Autodesk Inventor part; units mm, degrees
ref_plane "YZ Plane" through (0, 0, 0) normal (1, 0, 0) x (0, 1, 0)
ref_plane "XZ Plane" through (0, 0, 0) normal (0, 1, 0) x (-1, 0, 0)
ref_plane "XY Plane" through (0, 0, 0) normal (0, 0, 1) x (1, 0, 0)
sketch "Esquisse1" plane through (0, 0, 0) normal (0, 1, 0) x (-1, 0, 0)
  line L0 (25, 0) -> (125, 0)
  line L1 (150, -25) -> (150, -260)
  line L2 (125, -285) -> (25, -285)
  line L3 (0, -260) -> (0, -25)
  line L4 (20, 0) -> (20, -10) construction
  line L5 (20, -10) -> (0, -10) construction
  line L6 (150, 0) -> (0, -285) construction
  line L7 (150, -285) -> (0, 0) construction
  line L8 (75, 0) -> (75, -285) construction
  line L9 (150, -142.5) -> (0, -142.5) construction
  line L10 (30, -10) -> (120, -10)
  line L11 (130, -20) -> (130, -265)
  line L12 (120, -275) -> (30, -275)
  line L13 (20, -265) -> (20, -20)
  line L14 (130, -275) -> (150, -275) construction
  line L15 (130, -275) -> (130, -285) construction
  arc A0 (120, -275) -> (130, -265) centre (120, -265) ccw
  arc A1 (20, -265) -> (30, -275) centre (30, -265) ccw
  arc A2 (30, -10) -> (20, -20) centre (30, -20) ccw
  arc A3 (130, -20) -> (120, -10) centre (120, -20) ccw
  arc A4 (25, 0) -> (0, -25) centre (25, -25) ccw
  arc A5 (150, -25) -> (125, 0) centre (125, -25) ccw
  arc A6 (125, -285) -> (150, -260) centre (125, -260) ccw
  arc A7 (0, -260) -> (25, -285) centre (25, -260) ccw
  point P0 (150, -10)
  point P1 (148, 0)
  point P2 (0, -10)
  point P3 (10, 0)
  point P4 (0, -283)
  point P5 (2, -285)
  point P6 (140, -285)
  point P7 (150, -283)
  dimension "d0" = 150
  dimension "d5" = 20
  dimension "d11" = 10
  dimension "d13" = 10
  dimension "d14" = 265
  dimension "d15" = 25
extrude "Extrusion1" add sketch "Esquisse1" along normal blind 6
properties part number "top" material "Bois (cerisier)"
Geometry check sheet. Reference: the model listing, model coordinates, mm. A direction names the side the tool comes from. Round coordinates to 2 decimals unless told otherwise and drop trailing zeros. Write each loop counter-clockwise with the first axis right and the second up, starting at its lowest first coordinate (ties: lowest second). Pieces come first, ordered by that corner, then holes. Notation, with made-up numbers: (63.25, 20.5) -> (111.25, 20.5) arc R36 ccw to (111.25, 59.5) -> close; hole circle Ø3 at (-37.75, -29.75). An arc over 180 degrees is marked (long way). Put each result on its own line as item: value.
1) Release check for a two-part mould opening along X. For faces 1 (the face through (-19, 0, -142)), 2 (the face through (-23.01, 2.96, -272.15)), 3 (the face through (-142.871, 2.958, -277.482)) record: pulls with the +X half, pulls with the -X half, needs draft (parallel to the pull), parting line crosses it, or undercut.
Recorded:
face 1: needs draft
face 2: undercut
face 3: pulls with the -X half
2) Depth check by flat-ended pin: P1, Ø1, axis at y = 3.5, z = -33.5, coming from the +X side. Enter the tip coordinate at first touch or a pass-through.
Recorded:
P1: stops at x = 0
3) Cross-section at C-C, the plane y = 4. Enter the section's corners in (x, z).
Recorded:
outline: (-150, -260) arc R25 ccw to (-125, -285) -> (-25, -285) arc R25 ccw to (0, -260) -> (0, -25) arc R25 ccw to (-25, 0) -> (-125, 0) arc R25 ccw to (-150, -25) -> close; hole (-130, -265) arc R10 ccw to (-120, -275) -> (-30, -275) arc R10 ccw to (-20, -265) -> (-20, -20) arc R10 ccw to (-30, -10) -> (-120, -10) arc R10 ccw to (-130, -20) -> close
4) Cross-section at A-A, the plane x = -117. Enter the section's corners in (y, z), plus the area to 3 significant figures.
Recorded:
outline: (0, -285) -> (6, -285) -> (6, -275) -> (0, -275) -> close; (0, -10) -> (6, -10) -> (6, 0) -> (0, 0) -> close
area: 120 mm2
5) Thickness scan on probe 1 along Z at (x, y) = (-102.5, 0.3); probe 2 along X at (y, z) = (1.25, -237); probe 3 along X at (y, z) = (5.15, -12.5). Record the ranges inside material, lowest first. Write a range as from..to.
Recorded:
probe 1: z = -285..-275, -10..0
probe 2: x = -150..-130, -20..0
probe 3: x = -146.65..-126.61, -23.39..-3.35
6) Access from +Z, -Z, +X, -X, +Y, -Y to the whole of each face (thin tool, end or side, straight path). Record for faces 4 (the face through (-74, 3, 0)), 5 (the face through (-127.15, 2.96, -271.99)).
Recorded:
face 4: +Z, +X, -X, +Y, -Y
face 5: +Y, -Y
7) Cross-section at B-B, the plane z = -240. Enter the section's corners in (x, y).
Recorded:
outline: (-150, 0) -> (-130, 0) -> (-130, 6) -> (-150, 6) -> close; (-20, 0) -> (0, 0) -> (0, 6) -> (-20, 6) -> close
